Verification items for the finished model (mm, model axes). A direction names the side the tool comes from. Coordinates: 2 decimals unless noted, no trailing zeros. Order: outer loops, then holes, each group sorted by start corner. A loop starts at its lowest first (then second) coordinate and runs counter-clockwise, first axis right, second up. Notation, with made-up numbers: (-26, 45.25) -> (-15, 45.25) arc R27 cw to (-15, 80.25) -> close; hole circle Ø6 at (9, 6.5). An arc over 180 degrees is marked (long way). Write item = value, one per line. Start each with the question number.
from build123d import *

# Parameters (mm, degrees)
SKETCH1_R           = 3.175
BOSS_EXTRUDE1_DEPTH = 6.35
FILLET1_R           = 3.175
FILLET2_R           = 3.175
FILLET3_R           = 3.175
FILLET4_R           = 3.175


with BuildPart() as part:
    # Sketch1 → Boss-Extrude1 (new body)
    with BuildSketch(Plane(origin=(0, 0, 0), x_dir=(1, 0, 0), z_dir=(0, 1, 0))):
        Polygon((63.5, -7.9375), (76.2, -7.9375), (76.2, 0), (0, 0), (0, -50.8), (76.2, -50.8), (76.2, -12.7), (69.85, -12.7), (69.85, -25.4), (6.35, -25.4), (6.35, -19.05), (63.5, -19.05), align=None)
        with Locations(Location((25.4, -44.45, 0), (0, 0, 270))):
            Circle(SKETCH1_R, mode=Mode.SUBTRACT)
        with Locations(Location((50.8, -44.45, 0), (0, 0, 270))):
            Circle(SKETCH1_R, mode=Mode.SUBTRACT)
    extrude(amount=BOSS_EXTRUDE1_DEPTH)

    # Fillet1
    fillet1_edges = [part.edges().sort_by_distance(p)[0] for p in [
        (6.35, 3.175, 19.05),
        (6.35, 3.175, 25.4),
    ]]
    fillet(fillet1_edges, radius=FILLET1_R - 0.0001)  # a hair under: the kernel refuses the full size

    # Fillet2
    fillet2_edges = [part.edges().sort_by_distance(p)[0] for p in [
        (76.2, 3.175, 50.8),
        (0, 3.175, 50.8),
        (0, 3.175, 0),
        (76.2, 3.175, 0),
    ]]
    fillet(fillet2_edges, radius=FILLET2_R)

    # Fillet3
    fillet3_edges = [part.edges().sort_by_distance(p)[0] for p in [
        (76.2, 3.175, 12.7),
        (76.2, 3.175, 7.9375),
        (63.5, 3.175, 7.9375),
        (63.5, 3.175, 19.05),
        (69.85, 3.175, 25.4),
    ]]
    fillet(fillet3_edges, radius=FILLET3_R)

    # Fillet4
    fillet4_edges = [part.edges().sort_by_distance(p)[0] for p in [
        (69.85, 3.175, 12.7),
    ]]
    fillet(fillet4_edges, radius=FILLET4_R - 0.0001)  # a hair under: the kernel refuses the full size


solid = part.part
Item 1: Section check B-B (z = 44.45). Record the boundary of the cut face in (x, y) (3 decimals), then the cut area to 3 significant figures.
Item 2: Gauge pin test, flat ends, axial feed: P1, Ø1, axis at x = 65.5, z = 11, coming from the -Y side; P2, Ø4, axis at x = 52.5, z = 12.5, coming from the -Y side. Record the tip position at first contact, or that the pin passes through.
Item 3: Tool access check on faces 1 (the flat face through (70, 3, 7.938)), 2 (the cylindrical face through (75.25, 3.22, 49.89)), 3 (the cylindrical face through (70.8, 3.22, 13.61)). Record the directions out of +Z, -Z, +X, -X, +Y, -Y that give a thin tool (end or side, any length) a straight path to the whole face; none if there is none.
Item 4: Section check D-D (z = 15). Record the boundary of the cut face in (x, y), then the cut area to 3 significant figures.
Item 5: Section check A-A (x = 57). Record the boundary of the cut face in (y, z).
Item 6: Mould release check, pull along X, two halves, no side actions. Record for faces 4 (the flat face through (35, 3, 19.05)), 5 (the flat face through (0, 3, 25)), 6 (the flat face through (38, 0, 31)): pulls with the +X half, pulls with the -X half, needs draft (parallel to the pull), parting line crosses it, or undercut.
Item 7: Section check C-C (y = 3). State how many separate pieces and enclosed holes the cut face has, then the cut area to 3 significant figures.
Item 8: Thickness scan on line 1 (X direction, y = 3.75, z = 44.45) (3 decimals); line 2 (Z direction, x = 50.5, y = 4); line 3 (X direction, y = 4, z = 46.5). Record the ranges inside material, lowest first.
Filled sheet:
q1.outline = (0, 0) -> (22.225, 0) -> (22.225, 6.35) -> (0, 6.35) -> close; (28.575, 0) -> (47.625, 0) -> (47.625, 6.35) -> (28.575, 6.35) -> close; (53.975, 0) -> (76.2, 0) -> (76.2, 6.35) -> (53.975, 6.35) -> close
q1.area = 403 mm^2
q2.P1 = through
q2.P2 = 0
q3.face_1 = +X, +Y, -Y
q3.face_2 = +Z, +X, +Y, -Y
q3.face_3 = +Y, -Y
q4.outline = (0, 0) -> (63.5, 0) -> (63.5, 6.35) -> (0, 6.35) -> close; (69.97, 0) -> (76.08, 0) -> (76.08, 6.35) -> (69.97, 6.35) -> close
q4.area = 442 mm^2
q5.outline = (0, 0) -> (6.35, 0) -> (6.35, 19.05) -> (0, 19.05) -> close; (0, 25.4) -> (6.35, 25.4) -> (6.35, 50.8) -> (0, 50.8) -> close
q6.face_4 = undercut
q6.face_5 = pulls with the -X half
q6.face_6 = needs draft
q7.separate_pieces = 1
q7.enclosed_holes = 2
q7.area = 3,290 mm^2
q8.line_1 = 0 to 22.225, 28.575 to 47.625, 53.975 to 76.2
q8.line_2 = 0 to 19.05, 25.4 to 41.29, 47.61 to 50.8
q8.line_3 = 0 to 22.98, 27.82 to 48.38, 53.22 to 76.2
